Source: three-view drawing plus pictorial views. Frame: mm from the lowest corner of the part. A direction names the side the tool comes from. Give positions to 0.01 mm unless a question says otherwise; leave off trailing zeros. Loops run counter-clockwise (first coordinate to the right, second up) from the corner with the lowest first, then second, coordinate; pieces in that order, holes last. Notation, with made-up numbers: (-11.75, 42) - (24.25, 42) arc R13 cw to (24.25, 55) - close; hole circle Ø3 at (27.25, 49.5). An arc over 180 degrees is marked (long way). Write each question's results on one line, items separated by ' | '. Start each with the question number.
(1) Cut plane D-D on x = 42.5. Return the cut outline in (y, z), then the cut area to 3 significant figures.
(2) Contact query for flat-ended pins moving along their axis: pin 1 (1 mm diameter, centred on x = 12.5, y = 1.5, fed in from -Z); pin 2 (3 mm diameter, centred on x = 25, z = 5, fed in from -Y); pin 3 (1.5 mm diameter, centred on y = 2, z = 12.5, fed in from +X); pin 4 (1 mm diameter, centred on x = 38, y = 8, fed in from +Z). Output: stop coordinate, or through.
(3) Cut plane C-C on x = 3.5. Return the cut outline in (y, z).
(4) Reachability of the marked faces 1 and 2 from +Z, -Z, +X, -X, +Y, -Y: full face, straight path, thin tool, end or side. Return the list, or none.
(5) Cut plane A-A on z = 7.5. Return the cut outline in (x, y).
(6) Material intervals for line 1 along X through (y, z) = (13.25, 8); line 2 along Z through (x, y) = (7, 7.25), sorted ascending. Write a range as [from, to].
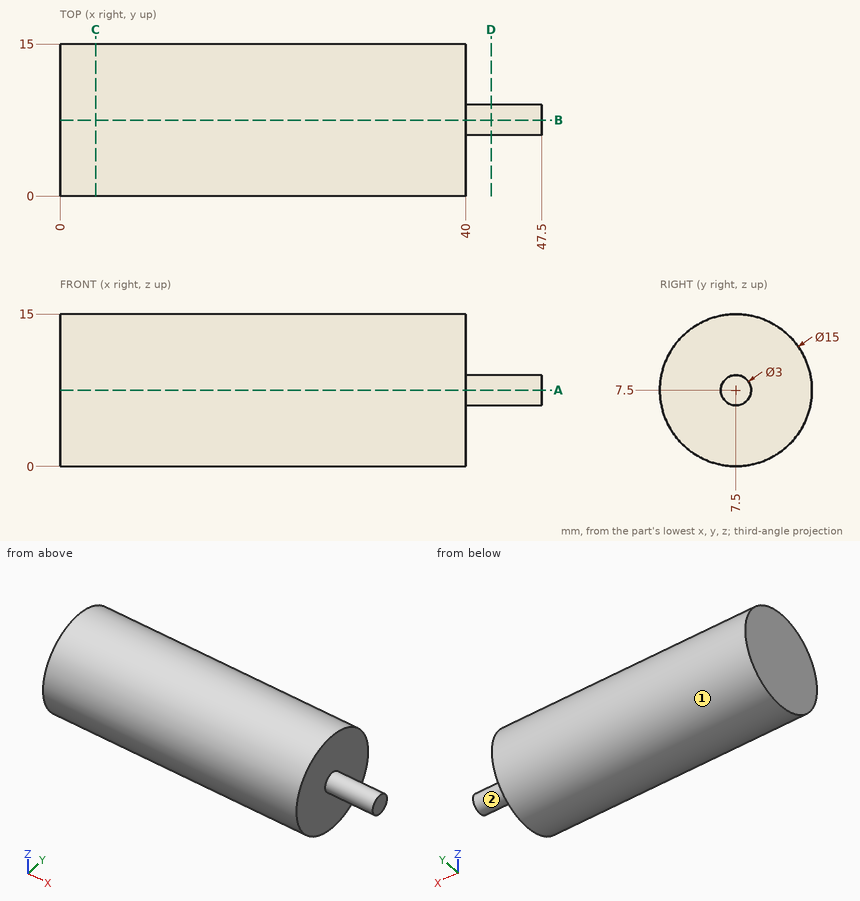
Ans:
1) outline: circle Ø3 at (7.5, 7.5) | area: 7.07 mm^2
2) pin 1: z = 2.4 | pin 2: y = 0.07 | pin 3: x = 40 | pin 4: z = 15
3) outline: circle Ø15 at (7.5, 7.5)
4) face 1: +X, -X | face 2: +X
5) outline: (0, 0) - (40, 0) - (40, 6) - (47.5, 6) - (47.5, 9) - (40, 9) - (40, 15) - (0, 15) - close
6) line 1: [0, 40] | line 2: [0, 15]
